Here's how the part is built. I have some questions about the finished solid (model axes, mm). A direction names the side the tool comes from. Round coordinates to 2 decimals unless told otherwise and drop trailing zeros. Loops run counter-clockwise (first coordinate to the right, second up) from the corner with the lowest first, then second, coordinate; pieces in that order, holes last. Notation, with made-up numbers: (-20, 71.5) -> (9, 71.5) arc R18 cw to (9, 82.5) -> close; hole circle Ø11 at (2.25, 55). An arc over 180 degrees is marked (long way). Use one line per item in the form item = value. Start each with the question number.
Item 1: If we section it at B-B (z = 259.5): Write out the boundary of the cut face in (x, y).
Item 2: I'm going to push flat-ended pins straight in: pin 1 Ø3 at (x, y) = (7.5, -10) entering from -Z; pin 2 Ø12 at (x, y) = (5, 18.5) entering from +Z; pin 3 Ø1.5 at (x, z) = (-1, 179.5) entering from -Y; pin 4 Ø6 at (x, z) = (3.5, -163.5) entering from +Y. Where does each tip first touch, or does it pass through?
Item 3: If we section it at A-A (z = 499.5): Write out the boundary of the cut face in (x, y), then the cut area to 3 significant figures.
Item 4: If I drill on L1, parallel to Z at x = -4.5, y = 5.5; L2, parallel to Z at x = 19, y = -8.5; L3, parallel to X at y = -3, z = -118, over which ranges is the centre line in solid material (lowest first)? Write a range as [from, to].
Item 5: For faces 1 (the face through (5, -5, -381)), 2 (the face through (-5.506, -24.796, 5.334)), 3 (the face through (-5, 5, 400.05)), 4 (the face through (-15.12, -11.59, 487.71)), 5 (the face through (0, 0, 577.85)), which set-ups out of +Z, -Z, +X, -X, +Y, -Y let a thin tool reach every point of the face, with its end or its side?
```python
from build123d import *

# Parameters (mm, degrees)
SKETCH1_R           = 6.35
BOSS_EXTRUDE1_DEPTH = 400.05
SKETCH1_3_R         = 25.4
SKETCH1_3_R_2       = 6.35
BOSS_EXTRUDE2_DEPTH = 381
BOSS_EXTRUDE3_START = 19.05
SKETCH3_R           = 19.05
BOSS_EXTRUDE3_DEPTH = 177.8


with BuildPart() as part:
    # Sketch1 → Boss-Extrude1 (new, symmetric)
    with BuildSketch(Plane.XY):
        with Locations(Location((0, 0, 0), (0, 0, 180))):
            Circle(SKETCH1_R)
    extrude(amount=BOSS_EXTRUDE1_DEPTH, both=True)

    # Sketch1_3 → Boss-Extrude2 (add, symmetric)
    with BuildSketch(Plane.XY):
        Circle(SKETCH1_3_R)
        with Locations(Location((0, 0, 0), (0, 0, 180))):
            Circle(SKETCH1_3_R_2, mode=Mode.SUBTRACT)
    extrude(amount=BOSS_EXTRUDE2_DEPTH, both=True)

    # Sketch3 → Boss-Extrude3 (add)
    with BuildSketch(Plane.XY.offset(381).offset(BOSS_EXTRUDE3_START)):
        Circle(SKETCH3_R)
    extrude(amount=BOSS_EXTRUDE3_DEPTH)


solid = part.part
```
Values found:
q1.outline = circle Ø50.8 at (0, 0)
q2.pin_1 = -381
q2.pin_2 = 577.85
q2.pin_3 = -25.4
q2.pin_4 = 25.4
q3.outline = circle Ø38.1 at (0, 0)
q3.area = 1,140 mm2
q4.L1 = [-381, 381], [400.05, 577.85]
q4.L2 = [-381, 381]
q4.L3 = [-25.22, 25.22]
q5.face_1 = -Z
q5.face_2 = +Z, -Z
q5.face_3 = none
q5.face_4 = +Z
q5.face_5 = +Z, +X, -X, +Y, -Y
